The listing builds one solid part. Answer for the finished solid, in the listing's coordinates (mm). A direction names the side the tool comes from. Round coordinates to 2 decimals unless told otherwise and drop trailing zeros. Write each loop counter-clockwise with the first axis right and the second up, starting at its lowest first coordinate (ties: lowest second). Pieces come first, ordered by that corner, then holes.
(1) Find the intervals of material crossed by probe 1 along X at (y, z) = (2.75, -2.5); probe 2 along Z at (x, y) = (48, -2); probe 3 along Y at (x, z) = (18.5, -1), in increasing order.
(2) The mould has two halves that part along Y. Classify faces 1 (the face through (-1.72, -1.08, 4.88)), 2 (the face through (-2.433, 1.014, 1.724)), 3 (the face through (0, 3.3, 0.1)): +Y half, -Y half, draft (parallel to the pull), parting line (faces both ways), or undercut.
(3) For faces 4 (the face through (-2.43, -0.99, 1.74)), 5 (the face through (29, -3, 0)), 6 (the face through (-4, -1, 2)), determine the directions among +Z, -Z, +X, -X, +Y, -Y from which every point of the face is accessible in a straight line to the end or side of a thin tool.
(4) A cutting plane is placed at A-A, the plane x = 44. Give the vertices of the cut face in (y, z), and give its area (3 significant figures).
(5) Each of these flat-tipped pins is pushed along its axis until it touches: pin 1 Ø4 at (x, z) = (9.5, -3) entering from -Y; pin 2 Ø3 at (x, y) = (13.5, 1) entering from +Z; pin 3 Ø0.7 at (x, z) = (-2, -0.5) entering from +Y; pin 4 Ø5 at (y, z) = (0.5, -1.5) entering from -X. Where does it stop, or does it pass through?
Autodesk Inventor part; units mm, degrees
ref_plane "Work Plane1" through (29, 0, 0) normal (0, -1, 0) x (1, 0, 0)
ref_plane "YZ Plane" through (0, 0, 0) normal (1, 0, 0) x (0, 1, 0)
ref_plane "XZ Plane" through (0, 0, 0) normal (0, 1, 0) x (-1, 0, 0)
sketch "Sketch1" plane through (0, 0, 0) normal (0, 0, 1) x (1, 0, 0)
  line L0 (0.3333, 0) -> (60, 0)
  line L1 (60, 0) -> (60, 3)
  line L2 (60, 3) -> (42, 3)
  line L3 (42, 3) -> (41.3865, 3)
  line L4 (41.3865, 3) -> (0, 3)
  line L5 (0, 3) -> (0, 5)
  line L6 (0, 5) -> (-4, 5)
  line L7 (-4, 5) -> (-4, 2.3094)
  line L8 (-4, 2.3094) -> (-1, 2.3094)
  line L9 (-1, 2.3094) -> (0.3333, 0)
  line L10 (-15.8, 0) -> (66.8, 0)
  line L11 (0, -1) -> (0, 6)
  line L12 (42, 3) -> (0, 3) construction
  dimension "d1" = 18
  dimension "d2" = 0.6136
  dimension "d3" = 4
  dimension "d4" = 3
  dimension "d5" = 60
  dimension "d6" = 6
  dimension "d7" = 6
  dimension "d8" = 4.6188
  dimension "d9" = 10
  dimension "d26" = 60
revolve "Body" add sketch "Sketch1" angle 360 about axis through (0.3333, 0, 0) along (1, 0, 0) contours L9 L11 L4 L3 L2 L1 L0 | L9 L8 L7 L6 L5 L11
sketch "Sketch2" plane through (-4, 0, 0) normal (-1, 0, 0) x (0, 0, 1)
  circle A0 centre (0, 0) radius 2.3094
  line L0 (0, -7) -> (0, 7)
  line L1 (-7, 0) -> (7, 0)
  line L2 (2.3094, 0) -> (1.1547, -2)
  line L3 (1.1547, -2) -> (-1.1547, -2)
  line L4 (-1.1547, -2) -> (-2.3094, 0)
  line L5 (-2.3094, 0) -> (-1.1547, 2)
  line L6 (-1.1547, 2) -> (1.1547, 2)
  line L7 (1.1547, 2) -> (2.3094, 0)
extrude "Slot" add sketch "Sketch2" against normal up to next contours L7 A0 | A0 L2 | L6 L0 A0 | A0 L0 L3 | L0 L6 A0 | A0 L3 L0 | L4 A0 | A0 L5
fillet "Fillet1" radius 0.6 1 edges at (-4, -5, 0)
thread "Thread"
chamfer "Chamfer1" distance 0.6135 distance2 0.6135 1 edges at (60, -3, 0) measured on face at (60, 1.5134, 0.7943)
ref_plane "Work Plane1" through (29, 0, 0) normal (0, -1, 0) x (1, 0, 0)
fillet "Fillet2" radius 0.1 1 edges at (0, -3, 0)
equation "\"d1\" = GEL"
equation "\"d3\" = KOH"
equation "\"d4\" = INTI"
equation "\"d6\" = GD"
equation "\"d7\" = BDM"
equation "\"d8\" = 1.1547 * SW"
equation "\"d9\" = KOD"
equation "\"d26\" = NLG"
equation "\"d30\" = R"
equation "\"d17\" = RR"
equation "\"d13\" = GEL"
equation "\"d15\" = -0.5 * SPD + 0.5 * GD"
equation "\"d16\" = GUL"
equation "\"GD\" = NND"
equation "\"NLG\" = 60"
equation "\"GEL\" = 18"
equation "\"KOD\" = 10"
equation "\"KOH\" = 4"
equation "\"INTI\" = 3"
equation "\"GAL\" = 0.61345 * PTC"
equation "\"GUL\" = 0.61345 * PTC"
equation "\"BDM\" = NND"
equation "\"SW\" = 4"
equation "\"RR\" = 0.6"
equation "\"SPD\" = NND - 1.2269 * PTC"
equation "\"R\" = 0.1"
equation "\"TOA\" = 30deg"
equation "\"GD1\" = THREADDIA - 1.2269 * PTC"
equation "\"THREADDIA\" = 6"
equation "\"FAWI\" = 45deg"
equation "\"ANG\" = 120deg"
equation "\"PTC\" = 1"
equation "\"NND\" = 6"
equation "\"E0\" = 1.155 * SW"
properties part number "DIN 7984 - M6 x 40" material "Steel, Mild"
Solutions:
1. probe 1: x = -4 to 0
1. probe 2: z = -2.24 to 2.24
1. probe 3: y = -2.83 to 2.83
2. face 1: parting line
2. face 2: undercut
2. face 3: draft
3. face 4: -X
3. face 5: +X
3. face 6: +Z, -Z, -X, +Y, -Y
4. outline: circle Ø6 at (0, 0)
4. area: 28.3 mm2
5. pin 1: stops at y = -2.83
5. pin 2: stops at z = 3
5. pin 3: stops at y = 5
5. pin 4: stops at x = -4
